Verification items for the finished model (mm, model axes). A direction names the side the tool comes from. Coordinates: 2 decimals unless noted, no trailing zeros. Order: outer loops, then holes, each group sorted by start corner. A loop starts at its lowest first (then second) coordinate and runs counter-clockwise, first axis right, second up. Notation, with made-up numbers: (58.25, 80.5) -> (90.25, 80.5) arc R15 cw to (90.25, 95.5) -> close; hole circle Ø5 at (0, -8). An arc over 180 degrees is marked (long way). Write each question's results on one line, items separated by ' | '. Start each with the question number.
(1) Cross-section at A-A on z = 0. Enter the section's corners in (x, y).
(2) Draft check along Y on faces 1 (the flat face through (22, 20, 22)), 2 (the flat face through (22, 0, 1)), 3 (the flat face through (0, 170, -1)). Enter one of: +Y half, -Y half, draft (parallel to the pull), parting line (faces both ways), or undercut.
(3) Thickness scan on probe 1 along X at (y, z) = (72, 0); probe 2 along X at (y, z) = (197.5, -1); probe 3 along Y at (x, z) = (-36, -29). Record the ranges inside material, lowest first. Write a range as [from, to].
(4) Set-up check for faces 4 (the flat face through (20, 270, 6)), 5 (the cylindrical face through (-19.524, 136.89, -4.336)), 6 (the cylindrical face through (-15.02, 9.86, -47.69)), 7 (the cylindrical face through (123.25, 203.195, 11.096)): record each of +Z, -Z, +X, -X, +Y, -Y from which the full face is reachable in a straight line by a thin tool's end or side.
(5) Cross-section at D-D on x = 230. Enter the section's corners in (y, z).
(6) Cross-section at B-B on y = 170. Enter the section's corners in (x, z).
(7) Go/stop test with flat-tipped pins: pin 1 (3 mm diameter, centred on x = -14.5, y = 230.5, fed in from -Z); pin 2 (12 mm diameter, centred on y = 231.5, z = -24.5, fed in from -X); pin 3 (10 mm diameter, centred on x = 69, z = 34.5, fed in from -Y). Record where each tip stops, or that it passes through.
(8) Cross-section at C-C on x = -25.5. Enter the section's corners in (y, z).
```python
from build123d import *

# Parameters (mm, degrees)
SKETCH4_R           = 20
CUT_EXTRUDE1_DEPTH  = 300
SKETCH5_R           = 35
BOSS_EXTRUDE1_DEPTH = 250


with BuildPart() as part:
    # Sketch1 → Revolve1 (revolve)
    with BuildSketch(Plane.XY, mode=Mode.PRIVATE) as revolve1_sk:
        Polygon((0, 0), (0, 270), (30, 270), (30, 20), (50, 20), (50, 0), align=None)
    revolve(revolve1_sk.sketch.rotate(Axis((0, 0, 0), (0, 1, 0)), 90), axis=Axis((0, 0, 0), (0, 1, 0)))

    # Sketch4 → Cut-Extrude1 (cut)
    with BuildSketch(Plane(origin=(0, 270, 0), x_dir=(1, 0, 0), z_dir=(0, 1, 0))):
        with Locations(Location((0, 0, 0), (0, 0, 270))):
            Circle(SKETCH4_R)
    extrude(amount=-CUT_EXTRUDE1_DEPTH, mode=Mode.SUBTRACT)

    # Sketch5 → Boss-Extrude1 (add)
    with BuildSketch(Plane(origin=(0, 0, 0), x_dir=(0, 0, -1), z_dir=(1, 0, 0))):
        with Locations(Location((0, 170, 0), (0, 0, 211.002719134))):
            Circle(SKETCH5_R)
    extrude(amount=BOSS_EXTRUDE1_DEPTH)


solid = part.part
```
Results are:
1) outline: (-50, 0) -> (-20, 0) -> (-20, 270) -> (-30, 270) -> (-30, 20) -> (-50, 20) -> close; (0, 135) -> (20, 135) -> (20, 0) -> (50, 0) -> (50, 20) -> (30, 20) -> (30, 135) -> (250, 135) -> (250, 205) -> (30, 205) -> (30, 270) -> (20, 270) -> (20, 205) -> (0, 205) -> close
2) face 1: undercut | face 2: -Y half | face 3: draft
3) probe 1: x = [-30, -20], [20, 30] | probe 2: x = [-29.98, -19.97], [0, 250] | probe 3: y = [0, 20]
4) face 4: +Z, -Z, +X, -X, +Y | face 5: none | face 6: -Y | face 7: +X
5) outline: circle Ø70 at (170, 0)
6) outline: (0, -35) -> (250, -35) -> (250, 35) -> (0, 35) -> (0, 30) arc R30 ccw to (0, -30) -> close; hole (0, -20) -> (0, 20) arc R20 ccw to start
7) pin 1: stops at z = -27.04 | pin 2: stops at x = -23.62 | pin 3: stops at y = 151.17
8) outline: (0, -43.01) -> (20, -43.01) -> (20, -15.8) -> (270, -15.8) -> (270, 15.8) -> (20, 15.8) -> (20, 43.01) -> (0, 43.01) -> close
